Verification items for the finished model (mm, model axes). Face numbers are marked on the shaded views. A direction names the side the tool comes from. Round coordinates to 2 decimals unless told otherwise and drop trailing zeros. Order: outer loops, then holes, each group sorted by start corner. A loop starts at its lowest first (then second) coordinate and runs counter-clockwise, first axis right, second up. Notation, with made-up numbers: (51, 75) -> (91, 75) arc R24 cw to (91, 114) -> close; hole circle Ø11 at (84, 77). An arc over 180 degrees is marked (long way). Put each result on its own line as item: value.
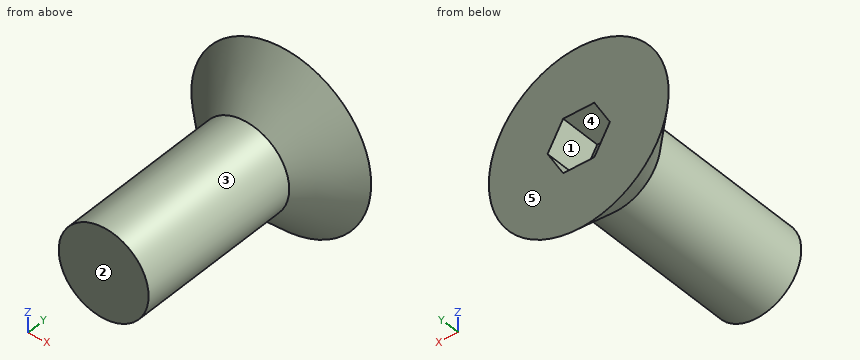
Autodesk Inventor part; units mm, degrees
ref_plane "YZ Plane" through (0, 0, 0) normal (1, 0, 0) x (0, 1, 0)
ref_plane "XZ Plane" through (0, 0, 0) normal (0, 1, 0) x (-1, 0, 0)
ref_plane "XY Plane" through (0, 0, 0) normal (0, 0, 1) x (1, 0, 0)
sketch "Head Revolution Profile" plane through (0, 0, 0) normal (0, 0, 1) x (1, 0, 0)
  line L0 (0, -5) -> (5, 0)
  line L1 (5, 0) -> (0, 0)
  line L2 (0, 0) -> (0, -5)
  dimension "d0" = 0
  dimension "d1" = 45
  dimension "d2" = 5
  dimension "d3" = 0
revolve "Head" add sketch "Head Revolution Profile" angle 360 about axis through (0, 0, 0) along (0, -1, 0)
sketch "Body Cross Section" plane through (0, 0, 0) normal (0, 1, 0) x (1, 0, 0)
  circle A0 centre (0, 0) radius 2.5
  point P0 (0, 0)
  dimension "d5" = 5
extrude "Body" add sketch "Body Cross Section" against normal blind 12
thread "Thread"
sketch "Key Socket Cutout Outline" plane through (0, 0, 0) normal (0, 1, 0) x (1, 0, 0)
  line L0 (0.866, 1.5) -> (1.7321, 0)
  line L1 (1.7321, 0) -> (0.866, -1.5)
  line L2 (0.866, -1.5) -> (-0.866, -1.5)
  line L3 (-0.866, -1.5) -> (-1.7321, 0)
  line L4 (-1.7321, 0) -> (-0.866, 1.5)
  line L5 (-0.866, 1.5) -> (0.866, 1.5)
  point P0 (0, 0)
  point P1 (0, 0)
  dimension "d10" = 3
extrude "Key Socket Cutout" cut sketch "Key Socket Cutout Outline" against normal blind 2.3
properties part number "SSK-M5-12-A4" material "Stainless Steel AISI 317"
Item 1: Section check B-B on x = 0. Record the boundary of the cut face in (y, z).
Check sheet entries:
outline: (-12, -2.5) -> (-2.5, -2.5) -> (0, -5) -> (0, -1.5) -> (-2.3, -1.5) -> (-2.3, 1.5) -> (0, 1.5) -> (0, 5) -> (-2.5, 2.5) -> (-12, 2.5) -> close
Item 2: Material ranges on L1, parallel to Z at x = -2, y = -6.5; L2, parallel to X at y = -1.75, z = 1.25, recorded low to high. Write a range as [from, to].
Check sheet entries:
L1: z = [-1.5, 1.5]
L2: x = [-3, -1.01], [1.01, 3]
Item 3: Tool access check on the marked faces 4 and 5. Record the directions out of +Z, -Z, +X, -X, +Y, -Y that give a thin tool (end or side, any length) a straight path to the whole face; none if there is none.
Check sheet entries:
face 4: +Y
face 5: +Z, -Z, +X, -X, +Y
Item 4: Release check for a two-part mould opening along Z. For the marked faces 1, 2 and 3 record: +Z half, -Z half, draft (parallel to the pull), parting line (faces both ways), or undercut.
Check sheet entries:
face 1: undercut
face 2: draft
face 3: parting line
Item 5: Gauge pin test, flat ends, axial feed: pin 1 Ø3 at (y, z) = (-4, -3.5) entering from -X; pin 2 Ø4 at (x, y) = (-4, -6) entering from -Z; pin 3 Ø1.9 at (x, y) = (0, -1) entering from -Z. Record the tip position at first contact, or that the pin passes through.
Check sheet entries:
pin 1: stops at x = -1.5
pin 2: stops at z = -1.5
pin 3: stops at z = -4.95
Item 6: Section check A-A on y = -2. Record the boundary of the cut face in (x, z).
Check sheet entries:
outline: circle Ø6 at (0, 0); hole (-1.73, 0) -> (-0.87, -1.5) -> (0.87, -1.5) -> (1.73, 0) -> (0.87, 1.5) -> (-0.87, 1.5) -> close
Item 7: Section check C-C on y = -3.5. Record the boundary of the cut face in (x, z).
Check sheet entries:
outline: circle Ø5 at (0, 0)
